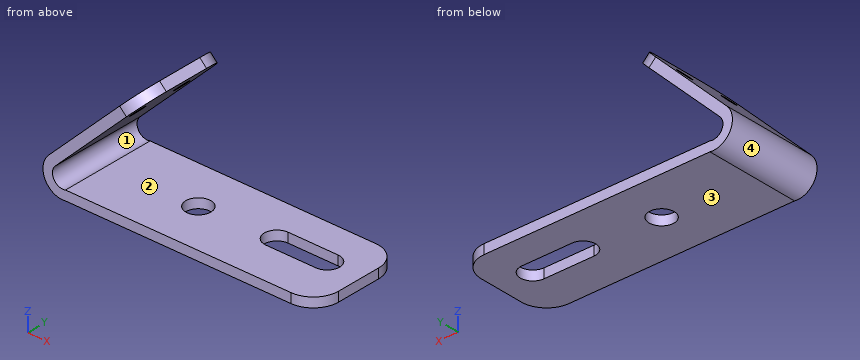
from build123d import *

# Parameters (mm, degrees)
F0_W     = 1270
F0_H     = 48.26
F1_DEPTH = 483.87
F2_R     = 127
F3_R     = 38.1
F4_DEPTH = 127
F5_R     = 63.5
F6_DEPTH = 50.8
F7_R     = 127


with BuildPart() as f1:
    # F0 (on Front) → F1 (new body)
    with BuildSketch(Plane.XZ):
        Rectangle(F0_W, F0_H)
        with BuildLine():
            ThreePointArc((-719.8287257737, 145.0706344887), (-738.4602241468, 29.8649791492), (-635, -24.13))
            Line((-635, -24.13), (-635, 24.13))
            ThreePointArc((-635, 24.13), (-693.8326988086, 47.9837165686), (-685.7037525136, 110.9456612286))
            Line((-685.7037525136, 110.9456612286), (-236.6909464602, 559.9584672821))
            Line((-236.6909464602, 559.9584672821), (-270.8159197202, 594.0834405421))
            Line((-270.8159197202, 594.0834405421), (-719.8287257737, 145.0706344887))
        make_face()
    extrude(amount=F1_DEPTH)

    # F2
    f2_edges = [f1.edges().sort_by_distance(p)[0] for p in [
        (-253.753433, -483.87, 577.020954),
        (-253.753433, 0, 577.020954),
    ]]
    fillet(f2_edges, radius=F2_R)

    # F3 (on face) → F4 (cut)
    with BuildSketch(Plane(origin=(-432.4496801312, 0, 432.4496801312), x_dir=(0, -1, 0), z_dir=(-0.7071067812, 0, 0.7071067812))):
        with Locations((114.3, 38.0846561105)):
            Circle(F3_R)
        with Locations((369.57, 38.0846561105)):
            Circle(F3_R)
    extrude(amount=-F4_DEPTH, mode=Mode.SUBTRACT)

    # F5 (on face) → F6 (cut)
    with BuildSketch(Plane.XY.offset(24.13)):
        with BuildLine():
            Line((203.4274212449, -284.3895672825), (457.4258095673, -284.3895672825))
            ThreePointArc((457.4258095673, -284.3895672825), (520.472977332, -220.663759187), (456.9725787551, -157.3895672825))
            Line((456.9725787551, -157.3895672825), (202.9741904327, -157.3895672825))
            ThreePointArc((202.9741904327, -157.3895672825), (139.4737860676, -221.1169928646), (203.4274212449, -284.3895672825))
        make_face()
        with Locations((-177.8, -240.2440756559)):
            Circle(F5_R)
    extrude(amount=-F6_DEPTH, mode=Mode.SUBTRACT)

    # F7
    f7_edges = [f1.edges().sort_by_distance(p)[0] for p in [
        (635, -483.87, 0),
        (635, 0, 0),
    ]]
    fillet(f7_edges, radius=F7_R)


solid = f1.part
Check sheet for the modelled part. Datum: model origin and axes. Units: mm. Face numbers are marked on the shaded views. Round coordinates to 2 decimals unless told otherwise and drop trailing zeros. Loops run counter-clockwise (first coordinate to the right, second up) from the corner with the lowest first, then second, coordinate; pieces in that order, holes last. Notation, with made-up numbers: M 20,-9.75 L 52,-9.75 A28 ccw 52,25.25 Z; hole C -27.5,-3.75 d4. An arc over 180 degrees is marked long. One line per item, written item: value.
(1) Release check for a two-part mould opening along Z. For the marked faces 1, 2, 3 and 4 record: +Z half, -Z half, draft (parallel to the pull), parting line (faces both ways), or undercut.
Computed values:
face 1: undercut
face 2: undercut
face 3: -Z half
face 4: parting line
(2) Depth check by flat-ended pin: pin 1 Ø1.5 at (y, z) = (-191.5, 509) entering from +X; pin 2 Ø1.5 at (y, z) = (-179.5, 302) entering from -X; pin 3 Ø1 at (x, y) = (413.5, -388.5) entering from -Z. Enter the tip coordinate at first touch or a pass-through.
Computed values:
pin 1: stops at x = -286.9
pin 2: stops at x = -563.65
pin 3: stops at z = -24.13
(3) Sectioned sample at A-A, the plane x = -177.8. Record the cut outline in (y, z).
Computed values:
outline: M -483.87,-24.13 L -303.74,-24.13 L -303.74,24.13 L -483.87,24.13 Z; M -176.74,-24.13 L 0,-24.13 L 0,24.13 L -176.74,24.13 Z
(4) Sectioned sample at D-D, the plane z = 240. Record the cut outline in (x, y).
Computed values:
outline: M -624.9,-483.87 L -556.65,-483.87 L -556.65,0 L -624.9,0 Z
(5) Thickness scan on line 1 (Y direction, x = -177, z = 7); line 2 (X direction, y = -363.5, z = 71); line 3 (Z direction, x = -328.5, y = -207). Record the ranges inside material, lowest first.
Computed values:
line 1: y = -483.87 to -303.74, -176.75 to 0
line 2: x = -748.97 to -700.83
line 3: z = -24.13 to 24.13, 468.15 to 536.4
(6) Sectioned sample at B-B, the plane y = -373. Record the cut outline in (x, z).
Computed values:
outline: M -719.83,145.07 A99.72 ccw -635,-24.13 L 633.97,-24.13 L 633.97,24.13 L -635,24.13 A51.97 cw -685.7,110.95 L -398.23,398.42 L -432.35,432.55 Z; M -378.69,486.21 L -344.56,452.09 L -237.42,559.23 L -271.54,593.36 Z
(7) Sectioned sample at C-C, the plane y = -104. Record the cut outline in (x, z).
Computed values:
outline: M -719.83,145.07 A99.72 ccw -635,-24.13 L 632.9,-24.13 L 632.9,24.13 L -635,24.13 A51.97 cw -685.7,110.95 L -397.33,399.32 L -431.46,433.44 Z; M -379.58,485.32 L -345.46,451.19 L -238.18,558.47 L -272.3,592.6 Z
